Autodesk Inventor part; units mm, degrees
ref_plane "YZ Plane" through (0, 0, 0) normal (1, 0, 0) x (0, 1, 0)
ref_plane "XZ Plane" through (0, 0, 0) normal (0, 1, 0) x (-1, 0, 0)
ref_plane "XY Plane" through (0, 0, 0) normal (0, 0, 1) x (1, 0, 0)
sketch "Sketch1" plane through (0, 0, 0) normal (0, 0, 1) x (1, 0, 0)
  line L0 (-6.6675, 0) -> (6.6675, 0)
  line L1 (0, -6.35) -> (0, 4.7625)
  line L2 (-3.175, 3.175) -> (-3.175, -3.175)
  line L3 (-3.175, -3.175) -> (3.175, -3.175)
  line L4 (3.175, -3.175) -> (3.175, 3.175)
  line L5 (4.7625, 3.175) -> (4.7625, -4.7625)
  line L6 (4.7625, -4.7625) -> (-4.7625, -4.7625)
  line L7 (-4.7625, -4.7625) -> (-4.7625, 3.175)
  line L8 (-3.175, 3.175) -> (-4.7625, 3.175)
  line L9 (3.175, 3.175) -> (4.7625, 3.175)
  point P0 (0, 0)
  point P1 (0, -3.175)
  point P2 (-3.175, 0)
  dimension "d0" = 1.5875
  dimension "d1" = 6.35
  dimension "d2" = 6.35
extrude "Extrusion1" add sketch "Sketch1" along normal mid plane 257.175 contours L7 L8 L2 L0 | L0 L2 L3 L1 L6 L7 | L1 L3 L4 L0 L5 L6 | L4 L9 L5 L0
sketch "Sketch2" plane through (4.7625, -4.7625, 128.5875) normal (1, 0, 0) x (0, 0, -1)
  line L0 (0, 7.9375) -> (0, 0)
  line L1 (0, 0) -> (257.175, 0)
  line L2 (0, 7.9375) -> (257.175, 7.9375)
  line L3 (0, 0) -> (7.9375, 7.9375)
  line L4 (7.9375, 7.9375) -> (0, 7.9375)
  line L5 (0, 7.9375) -> (0, 0)
  line L6 (128.5875, 7.9375) -> (128.5875, 0) construction
  line L7 (257.175, 7.9375) -> (257.175, 0)
  line L8 (257.175, 0) -> (249.2375, 7.9375)
  line L9 (257.175, 7.9375) -> (249.2375, 7.9375)
  line L10 (7.9375, 7.9375) -> (0, 7.9375)
  point P0 (128.5875, 4.7625)
  dimension "d5" = 45
extrude "Extrusion2" cut sketch "Sketch2" against normal through all contours L2 L3 L0 | L8 L2 L7
sketch "Sketch4" plane through (-4.7625, -4.7625, 128.5875) normal (0, -1, 0) x (1, 0, 0)
  circle A0 centre (4.7625, -103.1875) radius 1.5875
  circle A1 centre (4.7625, -153.9875) radius 1.5875
  point P0 (4.7625, -128.5875)
  dimension "d12" = 3.175
  dimension "d13" = 25.4
  dimension "d14" = 25.4
extrude "Extrusion4" add sketch "Sketch4" along normal blind 1.5875
properties part number "c-channel template" material "Aluminum-6061"
Verification items for the finished model (mm, model axes). A direction names the side the tool comes from. Give positions to 0.01 mm unless a question says otherwise; leave off trailing zeros. Write each loop counter-clockwise with the first axis right and the second up, starting at its lowest first coordinate (ties: lowest second). Pieces come first, ordered by that corner, then holes. Notation, with made-up numbers: M 82.5,60.25 L 87.5,60.25 A26 ccw 87.5,92.25 Z; hole C 30,88.25 d6. An arc over 180 degrees is marked long. One line per question, with ' | ' between items.
1) Thickness scan on line 1 along X through (y, z) = (2.5, 25.5) (1 decimal); line 2 along Y through (x, z) = (-0.5, 49) (1 decimal); line 3 along Y through (x, z) = (4, -40) (1 decimal). Record the ranges inside material, lowest first. Write a range as [from, to].
Result:
line 1: x = [-4.8, -3.2], [3.2, 4.8] | line 2: y = [-4.8, -3.2] | line 3: y = [-4.8, 3.2]
2) Mould release check, pull along X, two halves, no side actions. Record for faces 3 (the flat face through (4.762, -1, -2)), 4 (the flat face through (0, -4.762, -2)), 5 (the flat face through (3.175, 0, -2)): released by +X, released by -X, zero draft, split by the parting line, or undercut.
Result:
face 3: released by +X | face 4: zero draft | face 5: undercut
3) Section check B-B on y = 1.5. Enter the section's corners in (x, z) (1 decimal), plus the area to 3 significant figures.
Result:
outline: M -4.8,-122.3 L -3.2,-122.3 L -3.2,122.3 L -4.8,122.3 Z; M 3.2,-122.3 L 4.8,-122.3 L 4.8,122.3 L 3.2,122.3 Z | area: 777 mm2
4) Section check A-A on z = -64.5. Enter the section's corners in (x, y) (1 decimal).
Result:
outline: M -4.8,-4.8 L 4.8,-4.8 L 4.8,3.2 L 3.2,3.2 L 3.2,-3.2 L -3.2,-3.2 L -3.2,3.2 L -4.8,3.2 Z
5) Set-up check for faces 1 (the flat face through (1.125, -3.495, 127.32)), 2 (the flat face through (0, -3.175, -2)): record each of +Z, -Z, +X, -X, +Y, -Y from which the full face is reachable in a straight line by a thin tool's end or side.
Result:
face 1: +Z, +X, -X, +Y | face 2: +Z, -Z, +Y
6) Gauge pin test, flat ends, axial feed: pin 1 Ø2 at (x, z) = (2.5, 71) entering from -Y; pin 2 Ø5 at (x, z) = (0.5, 33.5) entering from +Y (3 decimals); pin 3 Ø1.5 at (x, y) = (0, -3.5) entering from +Z (3 decimals). Record the tip position at first contact, or that the pin passes through.
Result:
pin 1: stops at y = -4.76 | pin 2: stops at y = -3.175 | pin 3: stops at z = 128.075
